Study the drawing (mm; zero at the part's minimum x, y, z) and answer. A direction names the side the tool comes from. Coordinates: 2 decimals unless noted, no trailing zeros. Loops run counter-clockwise (first coordinate to the right, second up) from the corner with the lowest first, then second, coordinate; pieces in that order, holes last. Notation, with made-up numbers: (24.5, 22.25) -> (39.5, 22.25) arc R25 cw to (39.5, 36.25) -> close; hole circle Ø3 at (38.25, -29.75). An arc over 180 degrees is marked (long way). One line per question, with ' | ' between items. Start each with the question number.
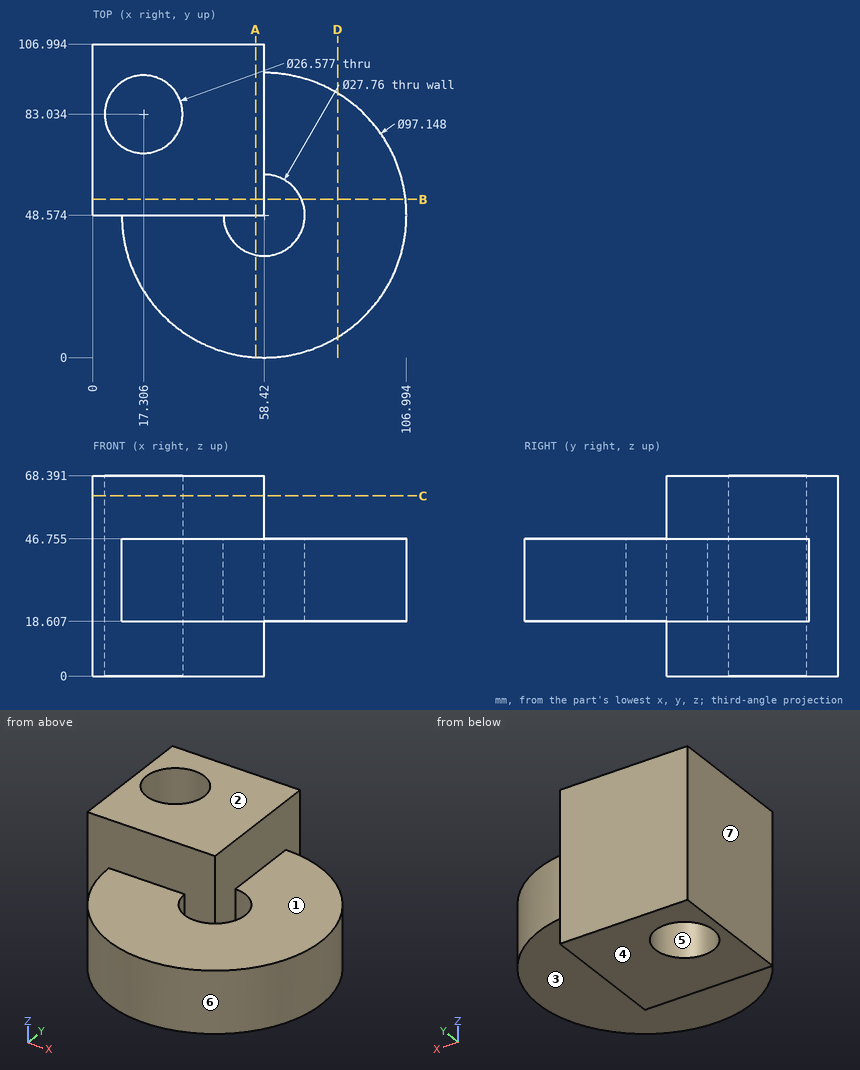
(1) Section A-A on x = 55.5 is taken. Write down the section's boundary in (y, z) (1 decimal).
(2) Section D-D on x = 83.5 is taken. Write down the section's boundary in (y, z) (1 decimal).
(3) Section B-B on y = 54 is taken. Write down the section's boundary in (x, z) (1 decimal), plus the area to 3 significant figures.
(4) Section C-C on z = 61.5 is taken. Write down the section's boundary in (x, y) (1 decimal).
(5) Each of these flat-tipped pins is pushed along its axis until it touches: pin 1 Ø6 at (y, z) = (12, 30.5) entering from +X; pin 2 Ø6 at (x, z) = (94.5, 23) entering from +Y; pin 3 Ø1 at (x, z) = (18, 37) entering from -Y; pin 4 Ø25 at (x, y) = (58.42, 48.57) entering from -Z. Where does it stop, or does it pass through?
(6) Determine the mould class of the marked faces 4, 5, 6 and 7 for opening direction X: +X half, -X half, draft (parallel to the pull), parting line (faces both ways), or undercut.
(7) Find the intervals of material crossed by probe 1 along Z at (x, y) = (57, 17) (1 decimal); probe 2 along Y at (x, z) = (20, 48.5) (1 decimal); probe 3 along X at (y, z) = (63.5, 3), in increasing order. Write a range as from..to.
(8) A tool of negligible diameter and unlimited length cuts with its end or side. For the marked faces 1, 2 and 3, from which of +Z, -Z, +X, -X, +Y, -Y can it reach the whole face along a straight path? Write none if from no direction.
Working result:
1) outline: (0.1, 18.6) -> (35, 18.6) -> (35, 46.8) -> (0.1, 46.8) -> close; (48.6, 0) -> (107, 0) -> (107, 68.4) -> (48.6, 68.4) -> close
2) outline: (7, 18.6) -> (90.2, 18.6) -> (90.2, 46.8) -> (7, 46.8) -> close
3) outline: (0, 0) -> (58.4, 0) -> (58.4, 68.4) -> (0, 68.4) -> close; (71.2, 18.6) -> (106.7, 18.6) -> (106.7, 46.8) -> (71.2, 46.8) -> close | area: 4,990 mm2
4) outline: (0, 48.6) -> (58.4, 48.6) -> (58.4, 107) -> (0, 107) -> close; hole circle Ø26.6 at (17.3, 83)
5) pin 1: stops at x = 93.52 | pin 2: stops at y = 84.14 | pin 3: stops at y = 20.9 | pin 4: stops at z = 0
6) face 4: draft | face 5: undercut | face 6: parting line | face 7: -X half
7) probe 1: z = 18.6..46.8 | probe 2: y = 48.6..70, 96..107 | probe 3: x = 0..58.42
8) face 1: +Z, +X, -Y | face 2: +Z, +X, -X, +Y, -Y | face 3: -Z, +X, -Y
